Print and shaded views of the part. All mm, measured from the part's lowest x, y and z. Round coordinates to 2 decimals unless told otherwise and drop trailing zeros. Write each loop counter-clockwise with the first axis right and the second up, starting at its lowest first coordinate (ties: lowest second). Pieces come first, ordered by that corner, then holes.
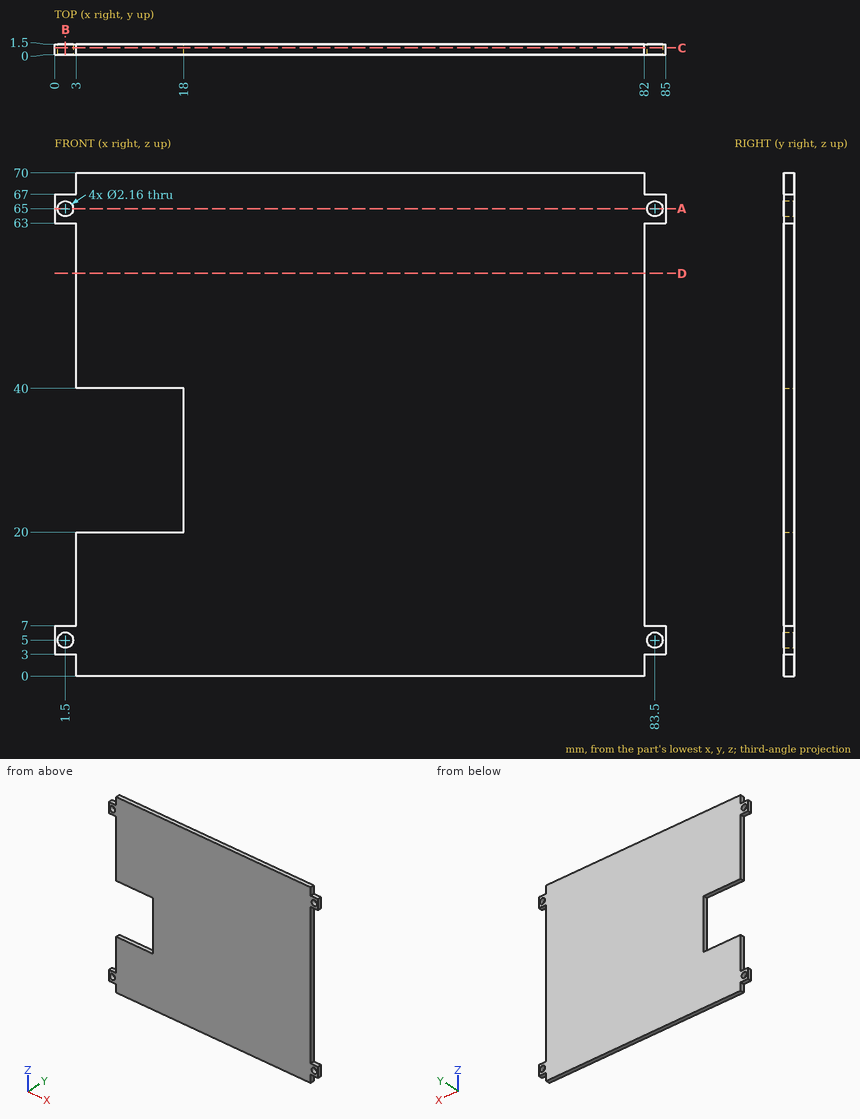
1) Pin check, flat tip, straight feed: pin 1 Ø0.8 at (x, y) = (2, 1) entering from +Z. Stop position of the tip, or through.
Results:
pin 1: stops at z = 67
2) Slice it at A-A (z = 65). Write the cut outline in (x, y).
Results:
outline: (0, 0) - (0.42, 0) - (0.42, 1.5) - (0, 1.5) - close; (2.58, 0) - (82.42, 0) - (82.42, 1.5) - (2.58, 1.5) - close; (84.58, 0) - (85, 0) - (85, 1.5) - (84.58, 1.5) - close
3) Slice it at B-B (x = 1.5). Write the cut outline in (y, z).
Results:
outline: (0, 3) - (1.5, 3) - (1.5, 3.92) - (0, 3.92) - close; (0, 6.08) - (1.5, 6.08) - (1.5, 7) - (0, 7) - close; (0, 63) - (1.5, 63) - (1.5, 63.92) - (0, 63.92) - close; (0, 66.08) - (1.5, 66.08) - (1.5, 67) - (0, 67) - close
4) Slice it at C-C (y = 0.95). Write the cut outline in (x, z), plus the area to 3 significant figures.
Results:
outline: (0, 3) - (3, 3) - (3, 0) - (82, 0) - (82, 3) - (85, 3) - (85, 7) - (82, 7) - (82, 63) - (85, 63) - (85, 67) - (82, 67) - (82, 70) - (3, 70) - (3, 67) - (0, 67) - (0, 63) - (3, 63) - (3, 40) - (18, 40) - (18, 20) - (3, 20) - (3, 7) - (0, 7) - close; hole circle Ø2.16 at (1.5, 5); hole circle Ø2.16 at (1.5, 65); hole circle Ø2.16 at (83.5, 5); hole circle Ø2.16 at (83.5, 65)
area: 5,260 mm2
5) Wall check: L1, parallel to X at y = 0.8, z = 65; L2, parallel to Z at x = 83.5, y = 1; L3, parallel to X at y = 0.9, z = 17. Give the ranges that are in metal, low to high.
Results:
L1: x = 0 to 0.42, 2.58 to 82.42, 84.58 to 85
L2: z = 3 to 3.92, 6.08 to 7, 63 to 63.92, 66.08 to 67
L3: x = 3 to 82
6) Slice it at D-D (z = 56). Write the cut outline in (x, y), plus the area to 4 significant figures.
Results:
outline: (3, 0) - (82, 0) - (82, 1.5) - (3, 1.5) - close
area: 118.5 mm2
